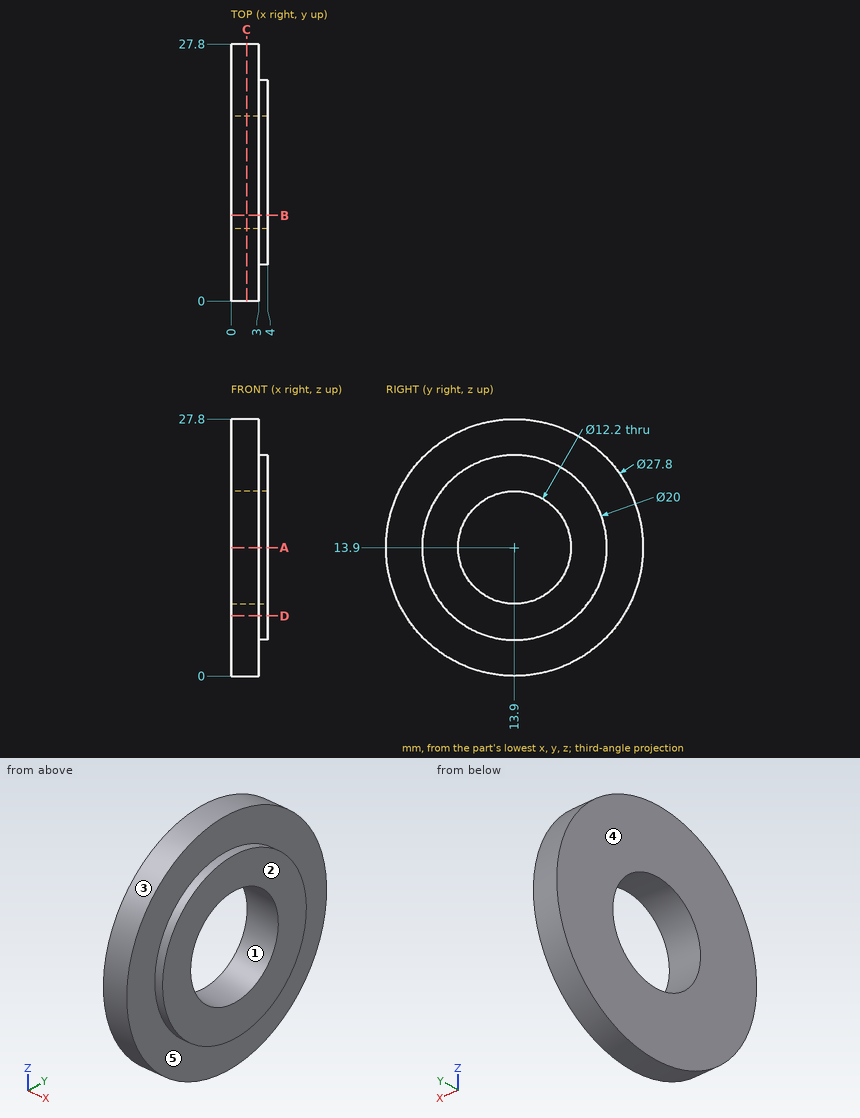
The drawing under review shows one solid part. Ordinate dimensions are in mm from its lowest x, y, z. A direction names the side the tool comes from. Round coordinates to 2 decimals unless told otherwise and drop trailing zeros. Loops run counter-clockwise (first coordinate to the right, second up) from the corner with the lowest first, then second, coordinate; pieces in that order, holes last. Notation, with made-up numbers: (60.25, 40.5) - (83.25, 40.5) arc R19 cw to (83.25, 64.5) - close; hole circle Ø7 at (-32.75, -9). An arc over 180 degrees is marked (long way). Use a Markdown table: item, result. Add a question column.
Q1. The part is to be moulded in two halves that separate along Z. For the marked faces 1, 2 and 3, say which applies: pulls with the +Z half, pulls with the -Z half, needs draft (parallel to the pull), parting line crosses it, or undercut.
Q2. Add section D-D (z = 6.5). State the section outline as (x, y) points, plus the area to 3 significant figures.
Q3. Add section C-C (x = 1.7). State the section outline as (y, z) points.
Q4. Machinability: for the marked faces 4 and 5, which of the approach directions +Z, -Z, +X, -X, +Y, -Y give a long, thin tool a straight path to every point of the face, cutting with its end or side? Answer none if there is none.
Q5. Add section A-A (z = 13.9). State the section outline as (x, y) points, plus the area to 3 significant figures.
Q6. Add section B-B (y = 9.25). State the section outline as (x, z) points.
Q7. Insertion check: pin 1 Ø10 at (y, z) = (13.9, 13.9) entering from +X; pin 2 Ø8 at (y, z) = (9, 24) entering from +X; pin 3 Ø1.5 at (x, z) = (2.5, 23.5) entering from -Y; pin 4 Ø2 at (x, z) = (2, 12.5) entering from +Y. Each pin has a flat end and moves straight along its axis. Give the tip position at first contact, or say it passes through.
Q8. For probe 1 along Z at (x, y) = (2, 13.9); probe 2 along X at (y, z) = (4, 17), list the stretches that pass through material, from the lowest coordinate up.
Worked answers:
| question | item | result |
|---|---|---|
| 1 | face 1 | undercut |
| 1 | face 2 | needs draft |
| 1 | face 3 | parting line crosses it |
| 2 | outline | (0, 2.13) - (3, 2.13) - (3, 7.17) - (4, 7.17) - (4, 20.63) - (3, 20.63) - (3, 25.67) - (0, 25.67) - close |
| 2 | area | 84.1 mm² |
| 3 | outline | circle Ø27.8 at (13.9, 13.9); hole circle Ø12.2 at (13.9, 13.9) |
| 4 | face 4 | +Z, -Z, -X, +Y, -Y |
| 4 | face 5 | +X |
| 5 | outline | (0, 0) - (3, 0) - (3, 3.9) - (4, 3.9) - (4, 7.8) - (0, 7.8) - close; (0, 20) - (4, 20) - (4, 23.9) - (3, 23.9) - (3, 27.8) - (0, 27.8) - close |
| 5 | area | 54.6 mm² |
| 6 | outline | (0, 0.8) - (3, 0.8) - (3, 5.05) - (4, 5.05) - (4, 9.95) - (0, 9.95) - close; (0, 17.85) - (4, 17.85) - (4, 22.75) - (3, 22.75) - (3, 27) - (0, 27) - close |
| 7 | pin 1 | through |
| 7 | pin 2 | x = 4 |
| 7 | pin 3 | y = 3.18 |
| 7 | pin 4 | y = 27.79 |
| 8 | probe 1 | 0 to 7.8, 20 to 27.8 |
| 8 | probe 2 | 0 to 3 |
